For this review, take the finished solid that the model builds, in its own axes (mm). Face numbers are marked on the shaded views. Round coordinates to 2 decimals unless told otherwise and drop trailing zeros. Loops run counter-clockwise (first coordinate to the right, second up) from the corner with the lowest first, then second, coordinate; pieces in that order, holes last. Notation, with made-up numbers: (76, 46) -> (131, 46) arc R26 cw to (131, 82) -> close; hole circle Ø11 at (20, -22.5). An arc over 180 degrees is marked (long way). Write each question's results on one line, items separated by ' | '.
```python
from build123d import *

# Parameters (mm, degrees)
BOSS_EXTRUDE1_DEPTH     = 60
BOSS_EXTRUDE2_DEPTH     = 32
CUT_EXTRUDE1_DEPTH      = 19.002558
CUT_EXTRUDE1_DEPTH_BACK = 19.002558
SKETCH3_R               = 5
CUT_EXTRUDE2_DEPTH      = 6
FILLET1_R               = 2
SKETCH4_R               = 1
CUT_EXTRUDE6_DEPTH      = 16
CUT_EXTRUDE6_DEPTH_BACK = 1
CUT_EXTRUDE7_DEPTH      = 16
FILLET2_R               = 5
FILLET3_R               = 10
FILLET4_R               = 10
CHAMFER2_SIZE           = 0.8


with BuildPart() as part:
    # Sketch1 → Boss-Extrude1 (new body)
    with BuildSketch(Plane(origin=(0, 0, 0), x_dir=(1, 0, 0), z_dir=(0, 1, 0))):
        with BuildLine():
            Line((-6.630435, 0), (6.630435, 0))
            Line((6.630435, 0), (14.467024, 0))
            Line((14.467024, 0), (18.002558, -3.535534))
            Line((18.002558, -3.535534), (18.002558, -15))
            Line((18.002558, -15), (15.602558, -15))
            Line((15.602558, -15), (15.5, -12.651045))
            ThreePointArc((15.5, -12.651045), (13.039719, -7.221088), (7.507614, -5))
            Line((7.507614, -5), (-7.507614, -5))
            ThreePointArc((-7.507614, -5), (-13.039719, -7.221088), (-15.5, -12.651045))
            Line((-15.5, -12.651045), (-15.602558, -15))
            Line((-15.602558, -15), (-18.002558, -15))
            Line((-18.002558, -15), (-18.002558, -3.535534))
            Line((-18.002558, -3.535534), (-14.467024, 0))
            Line((-14.467024, 0), (-6.630435, 0))
        make_face()
    extrude(amount=BOSS_EXTRUDE1_DEPTH)

    # Sketch1<2> → Boss-Extrude2 (add)
    with BuildSketch(Plane(origin=(0, 0, 0), x_dir=(1, 0, 0), z_dir=(0, 1, 0))):
        with BuildLine():
            Line((-6.630435, 0), (6.630435, 0))
            Line((6.630435, 0), (14.467024, 0))
            Line((14.467024, 0), (18.002558, -3.535534))
            Line((18.002558, -3.535534), (18.002558, -15))
            Line((18.002558, -15), (15.602558, -15))
            Line((15.602558, -15), (15.5, -12.651045))
            ThreePointArc((15.5, -12.651045), (13.039719, -7.221088), (7.507614, -5))
            Line((7.507614, -5), (-7.507614, -5))
            ThreePointArc((-7.507614, -5), (-13.039719, -7.221088), (-15.5, -12.651045))
            Line((-15.5, -12.651045), (-15.602558, -15))
            Line((-15.602558, -15), (-18.002558, -15))
            Line((-18.002558, -15), (-18.002558, -3.535534))
            Line((-18.002558, -3.535534), (-14.467024, 0))
            Line((-14.467024, 0), (-6.630435, 0))
        make_face()
    extrude(amount=-BOSS_EXTRUDE2_DEPTH)

    # Sketch2 → Cut-Extrude1 (cut, two sides)
    with BuildSketch(Plane(origin=(0, 0, 0), x_dir=(0, 0, -1), z_dir=(1, 0, 0))) as cut_extrude1_sk:
        Polygon((-15, 0), (-5, -10), (-5, -32), (-15, -32), align=None)
    extrude(amount=CUT_EXTRUDE1_DEPTH, mode=Mode.SUBTRACT)
    extrude(cut_extrude1_sk.sketch, amount=-CUT_EXTRUDE1_DEPTH_BACK, mode=Mode.SUBTRACT)

    # Sketch3 → Cut-Extrude2 (cut, through all)
    with BuildSketch(Plane.XY.offset(5)):
        with Locations((0, -22)):
            Circle(SKETCH3_R)
        Polygon((18.002558, -10.818656), (18.002558, -32), (5.773503, -32), align=None)
        Polygon((-18.002558, -32), (-5.773503, -32), (-18.002558, -10.818656), align=None)
    extrude(amount=-CUT_EXTRUDE2_DEPTH, mode=Mode.SUBTRACT)

    # Fillet1
    fillet1_edges = [part.edges().sort_by_distance(p)[0] for p in [
        (-5, -22, 5),
    ]]
    fillet(fillet1_edges, radius=FILLET1_R)

    # Sketch4 → Cut-Extrude6 (cut, two sides)
    with BuildSketch(Plane.XY) as cut_extrude6_sk:
        with Locations((5.3, 52)):
            Circle(SKETCH4_R)
        with Locations((-5.3, 52)):
            Circle(SKETCH4_R)
        with Locations((-5.3, 8)):
            Circle(SKETCH4_R)
        with Locations((5.3, 8)):
            Circle(SKETCH4_R)
    extrude(amount=CUT_EXTRUDE6_DEPTH, mode=Mode.SUBTRACT)
    extrude(cut_extrude6_sk.sketch, amount=-CUT_EXTRUDE6_DEPTH_BACK, mode=Mode.SUBTRACT)

    # Sketch5 → Cut-Extrude7 (cut, through all)
    with BuildSketch(Plane.XY):
        with BuildLine():
            Line((-1.5, 5.5), (-1.5, 10.5))
            ThreePointArc((-1.5, 10.5), (0, 12), (1.5, 10.5))
            Line((1.5, 10.5), (1.5, 5.5))
            ThreePointArc((1.5, 5.5), (0, 4), (-1.5, 5.5))
        make_face()
    extrude(amount=CUT_EXTRUDE7_DEPTH, mode=Mode.SUBTRACT)

    # Fillet2
    fillet2_edges = [part.edges().sort_by_distance(p)[0] for p in [
        (16.802558, 60, 15),
        (-16.802558, 60, 15),
    ]]
    fillet(fillet2_edges, radius=FILLET2_R)

    # Fillet3
    fillet3_edges = [part.edges().sort_by_distance(p)[0] for p in [
        (-16.802558, 0, 15),
        (16.802558, 0, 15),
    ]]
    fillet(fillet3_edges, radius=FILLET3_R)

    # Fillet4
    fillet4_edges = [part.edges().sort_by_distance(p)[0] for p in [
        (-12.755086, -10, 5),
        (12.755086, -10, 5),
    ]]
    fillet(fillet4_edges, radius=FILLET4_R)

    # Chamfer2
    chamfer2_edges = [part.edges().sort_by_distance(p)[0] for p in [
        (18.002558, -8.812535, 6.538596),
        (18.002558, 60, 6.767767),
        (18.002558, -5, 10),
        (18.002558, 58.535534, 13.535534),
        (18.002558, 0.315301, 14.238795),
        (18.002558, 29.571068, 15),
        (-18.002558, -8.812535, 6.538596),
        (-18.002558, 60, 6.767767),
        (-18.002558, -5, 10),
        (-18.002558, 58.535534, 13.535534),
        (-18.002558, 0.315301, 14.238795),
        (-18.002558, 29.571068, 15),
    ]]
    chamfer(chamfer2_edges, length=CHAMFER2_SIZE)


solid = part.part
```
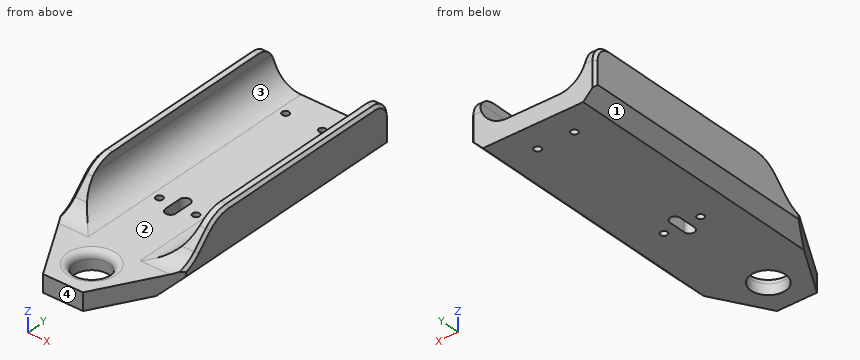
1. Consider section C-C (y = 8). State the section outline as (x, z) points, plus the area to 3 significant figures.
Values found:
outline: (-18, 3.54) -> (-14.47, 0) -> (-6.3, 0) -> (-6.3, 5) -> (-7.51, 5) arc R8 cw to (-15.5, 12.65) -> (-15.6, 15) -> (-17.2, 15) -> (-18, 14.2) -> close; (-4.3, 0) -> (-1.5, 0) -> (-1.5, 5) -> (-4.3, 5) -> close; (1.5, 0) -> (4.3, 0) -> (4.3, 5) -> (1.5, 5) -> close; (6.3, 0) -> (14.47, 0) -> (18, 3.54) -> (18, 14.2) -> (17.2, 15) -> (15.6, 15) -> (15.5, 12.65) arc R8 cw to (7.51, 5) -> (6.3, 5) -> close | area: 209 mm2
2. For pin 1 (1.2 mm diameter, centred on x = 5.3, y = 8, fed in from +Z); pin 2 (5 mm diameter, centred on x = -4.5, y = 40, fed in from +Z), all flat-tipped, find the tip position at first contact; note any pin that passes through.
Values found:
pin 1: passes through | pin 2: stops at z = 5
3. Consider section B-B (x = 0). State the section outline as (y, z) points.
Values found:
outline: (-32, 0) -> (-27, 0) -> (-27, 3) arc R2 ccw to (-29, 5) -> (-32, 5) -> close; (-17, 0) -> (4, 0) -> (4, 5) -> (-15, 5) arc R2 ccw to (-17, 3) -> close; (12, 0) -> (60, 0) -> (60, 5) -> (12, 5) -> close
4. Draft analysis for pull direction X (two halves, no side actions). For the marked faces 1, 2, 3 and 4, state which applies: released by +X, released by -X, zero draft, split by the parting line, or undercut.
Values found:
face 1: released by -X | face 2: undercut | face 3: undercut | face 4: zero draft
5. Consider section D-D (y = -22). State the section outline as (x, z) points, plus the area to 3 significant figures.
Values found:
outline: (-11.55, 0) -> (-5, 0) -> (-5, 3) arc R2 ccw to (-7, 5) -> (-11.55, 5) -> close; (5, 0) -> (11.55, 0) -> (11.55, 5) -> (7, 5) arc R2 ccw to (5, 3) -> close | area: 63.8 mm2
6. Consider section A-A (y = 52). State the section outline as (x, z) points, plus the area to 3 significant figures.
Values found:
outline: (-18, 3.54) -> (-14.47, 0) -> (-6.3, 0) -> (-6.3, 5) -> (-7.51, 5) arc R8 cw to (-15.5, 12.65) -> (-15.6, 15) -> (-17.2, 15) -> (-18, 14.2) -> close; (-4.3, 0) -> (4.3, 0) -> (4.3, 5) -> (-4.3, 5) -> close; (6.3, 0) -> (14.47, 0) -> (18, 3.54) -> (18, 14.2) -> (17.2, 15) -> (15.6, 15) -> (15.5, 12.65) arc R8 cw to (7.51, 5) -> (6.3, 5) -> close | area: 224 mm2
7. To check wall thickness, follow probe 1 along Y at (x, z) = (-5.3, 2.45); probe 2 along X at (y, z) = (8, 3.75); probe 3 along X at (y, z) = (52, 1.15). State the ranges of each line that lie inside material, in increasing order.
Values found:
probe 1: y = -32 to 7, 9 to 51, 53 to 60 | probe 2: x = -18 to -6.3, -4.3 to -1.5, 1.5 to 4.3, 6.3 to 18 | probe 3: x = -15.62 to -6.3, -4.3 to 4.3, 6.3 to 15.62
